Here's how the part is built. I have some questions about the finished solid (model axes, mm). Coordinates: 2 decimals unless noted, no trailing zeros. Order: outer loops, then holes, each group sorted by start corner. A loop starts at its lowest first (then second) coordinate and runs counter-clockwise, first axis right, second up. Notation, with made-up numbers: (-7.5, 15.25) - (8.5, 15.25) arc R19 cw to (8.5, 33.25) - close; hole circle Ø8 at (-8.5, 52). An arc over 180 degrees is marked (long way). Use one line per item in the form item = value. Start each with the question number.
from build123d import *

# Parameters (mm, degrees)
SKETCH1_R               = 609.6
SKETCH1_R_2             = 86.36
SKETCH1_R_3             = 34.925
BOSS_EXTRUDE1_DEPTH     = 12.7
CUT_EXTRUDE1_DEPTH      = 863.198126883
CUT_EXTRUDE1_DEPTH_BACK = 3.175


with BuildPart() as part:
    # Sketch1 → Boss-Extrude1 (new body)
    with BuildSketch(Plane.XY):
        with Locations(Location((0, 0, 0), (0, 0, 180))):
            Circle(SKETCH1_R)
        with Locations(Location((0, 508, 0), (0, 0, 180))):
            Circle(SKETCH1_R_2, mode=Mode.SUBTRACT)
        with Locations(Location((254, 439.940905122, 0), (0, 0, 180))):
            Circle(SKETCH1_R_2, mode=Mode.SUBTRACT)
        with Locations(Location((439.940905123, 254, 0), (0, 0, 180))):
            Circle(SKETCH1_R_2, mode=Mode.SUBTRACT)
        with Locations(Location((508, 0, 0), (0, 0, 180))):
            Circle(SKETCH1_R_2, mode=Mode.SUBTRACT)
        with Locations(Location((439.940905123, -254, 0), (0, 0, 180))):
            Circle(SKETCH1_R_2, mode=Mode.SUBTRACT)
        with Locations(Location((254, -439.940905122, 0), (0, 0, 180))):
            Circle(SKETCH1_R_2, mode=Mode.SUBTRACT)
        with Locations(Location((0, -508, 0), (0, 0, 180))):
            Circle(SKETCH1_R_2, mode=Mode.SUBTRACT)
        with Locations(Location((-254, -439.940905123, 0), (0, 0, 180))):
            Circle(SKETCH1_R_2, mode=Mode.SUBTRACT)
        with Locations(Location((-439.940905122, -254, 0), (0, 0, 180))):
            Circle(SKETCH1_R_2, mode=Mode.SUBTRACT)
        with Locations(Location((-508, 0, 0), (0, 0, 180))):
            Circle(SKETCH1_R_2, mode=Mode.SUBTRACT)
        with Locations(Location((-439.940905122, 254, 0), (0, 0, 180))):
            Circle(SKETCH1_R_2, mode=Mode.SUBTRACT)
        with Locations(Location((-254, 439.940905122, 0), (0, 0, 180))):
            Circle(SKETCH1_R_2, mode=Mode.SUBTRACT)
        with Locations(Location((0, 0, 0), (0, 0, 180))):
            Circle(SKETCH1_R_3, mode=Mode.SUBTRACT)
        Polygon((-263.817141205, 187.315483827), (-62.758262665, 187.315483827), (-62.758262665, 87.367139582), (-98.786154196, 87.367139582), (0, -145.651965314), (98.786154196, 87.367139582), (62.758262665, 87.367139582), (62.758262665, 187.315483827), (263.817141205, 187.315483827), (263.817141205, 87.367139582), (228.547895375, 87.367139582), (41.969279032, -352.738890732), (-41.969279032, -352.738890732), (-228.547895375, 87.367139582), (-263.817141205, 87.367139582), align=None, mode=Mode.SUBTRACT)
    extrude(amount=BOSS_EXTRUDE1_DEPTH)

    # Sketch2 → Cut-Extrude1 (cut, two sides: drawn at the far end of the back side and taken through both)
    with BuildSketch(Plane.XY.offset(12.7).offset(-CUT_EXTRUDE1_DEPTH_BACK)):
        Polygon((50.058262665, 74.667139582), (79.607989254, 74.667139582), (0, -113.1140586), (-79.607989254, 74.667139582), (-50.058262665, 74.667139582), (-50.058262665, 200.015483827), (-276.517141205, 200.015483827), (-276.517141205, 74.667139582), (-236.957980515, 74.667139582), (-50.379364172, -365.438890732), (50.379364172, -365.438890732), (236.957980515, 74.667139582), (276.517141205, 74.667139582), (276.517141205, 200.015483827), (50.058262665, 200.015483827), align=None)
        Polygon((-41.969279032, -352.738890732), (-228.547895375, 87.367139582), (-263.817141205, 87.367139582), (-263.817141205, 187.315483827), (-62.758262665, 187.315483827), (-62.758262665, 87.367139582), (-98.786154196, 87.367139582), (0, -145.651965314), (98.786154196, 87.367139582), (62.758262665, 87.367139582), (62.758262665, 187.315483827), (263.817141205, 187.315483827), (263.817141205, 87.367139582), (228.547895375, 87.367139582), (41.969279032, -352.738890732), align=None, mode=Mode.SUBTRACT)
    extrude(amount=CUT_EXTRUDE1_DEPTH + CUT_EXTRUDE1_DEPTH_BACK, mode=Mode.SUBTRACT)


solid = part.part
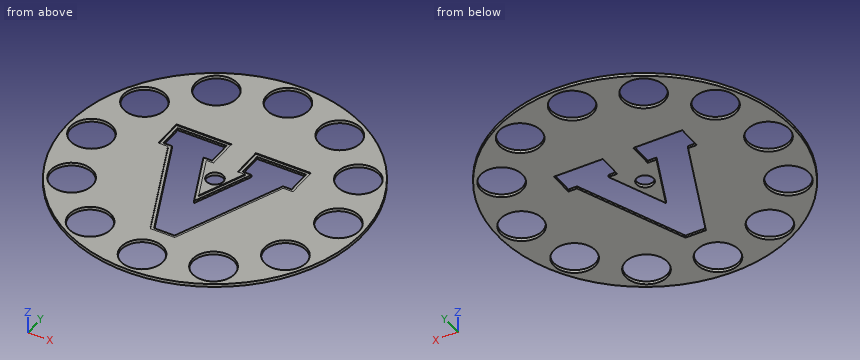
1) Suppose I cut it at B-B, the plane x = -394. List the corners of the cut face in (y, z) for me.
2) Suppose I cut it at A-A, the plane x = 501.5. List the corners of the cut face in (y, z) for me.
3) Suppose I cut it at D-D, the plane z = 7.5. Give the number of separate pieces and of enclosed holes in the cut face, then the cut area to 3 significant figures.
4) I need wall thicknesses on probe 1 along Y at (x, z) = (0, 2.5) (3 decimals); probe 2 along X at (y, z) = (-508, 8.5); probe 3 along X at (y, z) = (239, 4). Which ranges of each line are inside material? Lowest first, please. Write a range as [from, to].
5) Suppose I cut it at C-C, the plane y = 508. List the corners of the cut face in (x, z) for me, then the cut area to 3 significant figures.
6) For pin 1 (12 mm diameter, centred on x = 296.5, y = -6, fed in from -Z); pin 2 (3 mm diameter, centred on y = 130.5, z = 5.5, fed in from -X); pin 3 (1 mm diameter, centred on x = 168, z = 10.5, fed in from -Y); pin 4 (4 mm diameter, centred on x = 471.5, z = 9.5, fed in from +Y), each with a flat end and sliding along its axis, tell me the tip position at first contact or that it passes through.
From the geometry:
q1.outline = (-465.16, 0) - (-327.13, 0) - (-327.13, 12.7) - (-465.16, 12.7) - close; (-180.87, 0) - (180.87, 0) - (180.87, 12.7) - (-180.87, 12.7) - close; (327.13, 0) - (465.16, 0) - (465.16, 12.7) - (327.13, 12.7) - close
q2.outline = (-346.57, 0) - (-314.57, 0) - (-314.57, 12.7) - (-346.57, 12.7) - close; (-193.43, 0) - (-86.12, 0) - (-86.12, 12.7) - (-193.43, 12.7) - close; (86.12, 0) - (193.43, 0) - (193.43, 12.7) - (86.12, 12.7) - close; (314.57, 0) - (346.57, 0) - (346.57, 12.7) - (314.57, 12.7) - close
q3.separate_pieces = 1
q3.enclosed_holes = 14
q3.area = 746,000 mm2
q4.probe_1 = [-609.6, -594.36], [-421.64, -352.739], [-145.652, -34.925], [34.925, 421.64], [594.36, 609.6]
q4.probe_2 = [-336.97, -307.16], [-200.84, -86.36], [86.36, 200.84], [307.16, 336.97]
q4.probe_3 = [-560.8, -524.99], [-354.89, 354.89], [524.99, 560.8]
q5.outline = (-336.97, 0) - (-307.16, 0) - (-307.16, 12.7) - (-336.97, 12.7) - close; (-200.84, 0) - (-86.36, 0) - (-86.36, 12.7) - (-200.84, 12.7) - close; (86.36, 0) - (200.84, 0) - (200.84, 12.7) - (86.36, 12.7) - close; (307.16, 0) - (336.97, 0) - (336.97, 12.7) - (307.16, 12.7) - close
q5.area = 3,660 mm2
q6.pin_1 = 0
q6.pin_2 = -595.79
q6.pin_3 = -586.14
q6.pin_4 = 388.82
